Autodesk Inventor part; units mm, degrees
ref_plane "dummy_XY" through (0, 0, 0) normal (1, 0, 0) x (0, 0, -1)
ref_plane "dummy_YZ" through (0, 0, 0) normal (0, 0, -1) x (0, 1, 0)
ref_plane "dummy_ZX" through (0, 0, 0) normal (0, 1, 0) x (1, 0, 0)
sketch "Sketch_1" plane through (0, 0, 0) normal (1, 0, 0) x (0, 1, 0)
  line L0 (-22, 13) -> (-22.5, 12.5)
  line L1 (-22.5, 12.5) -> (-22.5, 2.25)
  line L2 (-22.5, 2.25) -> (-18.5, 2.25)
  line L3 (-18.5, 2.25) -> (-18.5, 1.9)
  arc A0 (-18.5, 1.9) -> (-18.3, 1.7) centre (-18.3, 1.9) ccw
  line L4 (-18.3, 1.7) -> (-17, 1.7)
  line L5 (-17, 1.7) -> (-16.5, 2.15)
  line L6 (-16.5, 2.15) -> (-14.7, 2.15)
  arc A1 (-13, 0.45) -> (-14.7, 2.15) centre (-14.7, 0.45) ccw
  line L7 (-13, 0.45) -> (-13, -0.45)
  arc A2 (-14.7, -2.15) -> (-13, -0.45) centre (-14.7, -0.45) ccw
  line L8 (-14.7, -2.15) -> (-16.5, -2.15)
  line L9 (-16.5, -2.15) -> (-17, -1.7)
  line L10 (-17, -1.7) -> (-18.3, -1.7)
  arc A3 (-18.3, -1.7) -> (-18.5, -1.9) centre (-18.3, -1.9) ccw
  line L11 (-18.5, -1.9) -> (-18.5, -2.25)
  line L12 (-18.5, -2.25) -> (-22.5, -2.25)
  line L13 (-22.5, -2.25) -> (-22.5, -12.5)
  line L14 (-22.5, -12.5) -> (-22, -13)
  line L15 (-22, -13) -> (22, -13)
  line L16 (22, -13) -> (22.5, -12.5)
  line L17 (22.5, -12.5) -> (22.5, -2.25)
  line L18 (22.5, -2.25) -> (18.5, -2.25)
  line L19 (18.5, -2.25) -> (18.5, -1.9)
  arc A4 (18.5, -1.9) -> (18.3, -1.7) centre (18.3, -1.9) ccw
  line L20 (18.3, -1.7) -> (17, -1.7)
  line L21 (17, -1.7) -> (16.5, -2.15)
  line L22 (16.5, -2.15) -> (14.7, -2.15)
  arc A5 (13, -0.45) -> (14.7, -2.15) centre (14.7, -0.45) ccw
  line L23 (13, -0.45) -> (13, 0.45)
  arc A6 (14.7, 2.15) -> (13, 0.45) centre (14.7, 0.45) ccw
  line L24 (14.7, 2.15) -> (16.5, 2.15)
  line L25 (16.5, 2.15) -> (17, 1.7)
  line L26 (17, 1.7) -> (18.3, 1.7)
  arc A7 (18.3, 1.7) -> (18.5, 1.9) centre (18.3, 1.9) ccw
  line L27 (18.5, 1.9) -> (18.5, 2.25)
  line L28 (18.5, 2.25) -> (22.5, 2.25)
  line L29 (22.5, 2.25) -> (22.5, 12.5)
  line L30 (22.5, 12.5) -> (22, 13)
  line L31 (22, 13) -> (-22, 13)
extrude "Extrusion1" add sketch "Sketch_1" along normal blind 50
sketch "Sketch2" plane through (50, 0, 0) normal (1, 0, 0) x (0, 0, -1)
  point P0 (0, 0)
hole "Hole1" at (50, 0, 0) direction (-1, 0, 0) diameter 22 depth 1.5
sketch "Sketch3" plane through (50, 0, 0) normal (1, 0, 0) x (0, 0, -1)
  point P0 (8, 17.5)
hole "Hole2" at (50, 17.5, -8) direction (-1, 0, 0) diameter 4 depth 4
sketch "Sketch_3" plane through (0, 0, 0) normal (0, 1, 0) x (-1, 0, 0)
  line L0 (0, 6.05) -> (-18.5, 6.05)
  line L1 (-18.5, 6.05) -> (-18.5, -6.05)
  line L2 (-18.5, -6.05) -> (0, -6.05)
  line L3 (0, -6.05) -> (0, 6.05)
extrude "Extrusion2" cut sketch "Sketch_3" along normal mid plane 60
sketch "Sketch5" plane through (50, 0, 0) normal (1, 0, 0) x (0, 0, -1)
  point P0 (8, -17.5)
hole "Hole3" at (50, -17.5, -8) direction (-1, 0, 0) diameter 4.134 depth 11 tip angle 120 countersink diameter 5 countersink angle 90
sketch "Sketch6" plane through (50, 0, 0) normal (1, 0, 0) x (0, 0, -1)
  point P0 (-8, 17.5)
hole "Hole4" at (50, 17.5, 8) direction (-1, 0, 0) diameter 4.134 depth 11 tip angle 120 countersink diameter 5 countersink angle 90
sketch "Sketch_6" plane through (0, 0, 6.5) normal (0, 0, 1) x (1, 0, 0)
  line L0 (25, 6.3066) -> (25, 22.5)
  line L1 (25, 22.5) -> (27.5, 22.5)
  line L2 (27.5, 22.5) -> (27.067, 22.067)
  line L3 (27.067, 22.067) -> (27.067, 15.5)
  line L4 (27.067, 15.5) -> (25.75, 14.7396)
  line L5 (25.75, 14.7396) -> (25.75, 6.7396)
  line L6 (25.75, 6.7396) -> (25, 6.3066)
  line L7 (25, 6.3066) -> (25, 22.5)
revolve "Revolution1" cut sketch "Sketch_6" angle 360 about axis through (25, 6.3066, 6.5) along (0, -1, 0)
thread "Thread1"
sketch "Sketch_7" plane through (0, 0, -6.5) normal (0, 0, 1) x (1, 0, 0)
  line L0 (42, 6.3066) -> (42, 22.5)
  line L1 (42, 22.5) -> (44.5, 22.5)
  line L2 (44.5, 22.5) -> (44.067, 22.067)
  line L3 (44.067, 22.067) -> (44.067, 15.5)
  line L4 (44.067, 15.5) -> (42.75, 14.7396)
  line L5 (42.75, 14.7396) -> (42.75, 6.7396)
  line L6 (42.75, 6.7396) -> (42, 6.3066)
  line L7 (42, 6.3066) -> (42, 22.5)
revolve "Revolution2" cut sketch "Sketch_7" angle 360 about axis through (42, 6.3066, -6.5) along (0, -1, 0)
thread "Thread2"
sketch "Sketch9" plane through (0, -22.5, 12.5) normal (0, -1, 0) x (1, 0, 0)
  point P0 (31, -4.5)
hole "Hole5" at (31, -22.5, 8) direction (0, 1, 0) diameter 4.134 depth 11 tip angle 120 countersink diameter 5 countersink angle 90
sketch "Sketch10" plane through (0, -22.5, -12.5) normal (0, -1, 0) x (1, 0, 0)
  point P0 (31, 4.5)
hole "Hole6" at (31, -22.5, -8) direction (0, 1, 0) diameter 4.134 depth 11 tip angle 120 countersink diameter 5 countersink angle 90
sketch "Sketch11" plane through (0, -22, -13) normal (0, 0, -1) x (-1, 0, 0)
  point P0 (-25, 7)
hole "Hole7" at (25, -15, -13) direction (0, 0, 1) diameter 4.134 depth 12 tip angle 120 countersink diameter 5 countersink angle 90
sketch "Sketch12" plane through (0, -22, -13) normal (0, 0, -1) x (-1, 0, 0)
  point P0 (-25, 37)
hole "Hole8" at (25, 15, -13) direction (0, 0, 1) diameter 4.134 depth 12 tip angle 120 countersink diameter 5 countersink angle 90
sketch "Sketch_14" plane through (0, 15, 0) normal (0, 1, 0) x (1, 0, 0)
  line L0 (10.5, -13) -> (10.5, 13)
  line L1 (10.5, 13) -> (12.7, 13)
  line L2 (12.7, 13) -> (12.5, 12.8)
  line L3 (12.5, 12.8) -> (12.5, -12.8)
  line L4 (12.5, -12.8) -> (12.7, -13)
  line L5 (12.7, -13) -> (10.5, -13)
  line L6 (10.5, -13) -> (10.5, 13)
revolve "Revolution3" cut sketch "Sketch_14" angle 360 about axis through (10.5, 15, 13) along (0, 0, 1)
sketch "Sketch_15" plane through (0, -15, 0) normal (0, 1, 0) x (1, 0, 0)
  line L0 (10.5, -13) -> (10.5, 13)
  line L1 (10.5, 13) -> (12.7, 13)
  line L2 (12.7, 13) -> (12.5, 12.8)
  line L3 (12.5, 12.8) -> (12.5, -12.8)
  line L4 (12.5, -12.8) -> (12.7, -13)
  line L5 (12.7, -13) -> (10.5, -13)
  line L6 (10.5, -13) -> (10.5, 13)
revolve "Revolution4" cut sketch "Sketch_15" angle 360 about axis through (10.5, -15, 13) along (0, 0, 1)
sketch "Sketch_20" plane through (10.5, 0, 0) normal (1, 0, 0) x (0, 0, -1)
  line L0 (-12.9, 15) -> (12.9, 15)
  line L1 (12.9, 15) -> (12.9, 13)
  line L2 (12.9, 13) -> (-12.9, 13)
  line L3 (-12.9, 13) -> (-12.9, 15)
  line L4 (-12.9, 15) -> (12.9, 15)
revolve "Revolution5" add sketch "Sketch_20" angle 360 about axis through (10.5, 15, 12.9) along (0, 0, 1)
sketch "Sketch_21" plane through (10.5, 0, 0) normal (1, 0, 0) x (0, 0, -1)
  line L0 (-12.9, -15) -> (12.9, -15)
  line L1 (12.9, -15) -> (12.9, -17)
  line L2 (12.9, -17) -> (-12.9, -17)
  line L3 (-12.9, -17) -> (-12.9, -15)
  line L4 (-12.9, -15) -> (12.9, -15)
revolve "Revolution6" add sketch "Sketch_21" angle 360 about axis through (10.5, -15, 12.9) along (0, 0, 1)
ref_plane "dummy_XY" through (0, 0, 0) normal (1, 0, 0) x (0, 0, -1)
ref_plane "dummy_YZ" through (0, 0, 0) normal (0, 0, -1) x (0, 1, 0)
ref_plane "dummy_ZX" through (0, 0, 0) normal (0, 1, 0) x (1, 0, 0)
ref_plane "grip_XY" through (10.5, 15, 0) normal (0, 0, 1) x (1, 0, 0)
ref_plane "grip_YZ" through (10.5, 15, 0) normal (1, 0, 0) x (0, 1, 0)
ref_plane "grip_ZX" through (10.5, 15, 0) normal (0, 1, 0) x (0, 0, 1)
ref_plane "grip1_XY" through (10.5, -15, 0) normal (0, 0, 1) x (1, 0, 0)
ref_plane "grip1_YZ" through (10.5, -15, 0) normal (1, 0, 0) x (0, 1, 0)
ref_plane "grip1_ZX" through (10.5, -15, 0) normal (0, 1, 0) x (0, 0, 1)
ref_plane "switch_XY" through (20.8, 13, 0) normal (-1, 0, 0) x (0, 0, -1)
ref_plane "switch_YZ" through (20.8, 13, 0) normal (0, 0, -1) x (0, -1, 0)
ref_plane "switch_ZX" through (20.8, 13, 0) normal (0, -1, 0) x (-1, 0, 0)
ref_plane "switch2_XY" through (26.1, -13, 0) normal (-1, 0, 0) x (0, 0, -1)
ref_plane "switch2_YZ" through (26.1, -13, 0) normal (0, 0, -1) x (0, -1, 0)
ref_plane "switch2_ZX" through (26.1, -13, 0) normal (0, -1, 0) x (-1, 0, 0)
properties part number "MCHA-20_(b)"
For this review, take the finished solid that the model builds, in its own axes (mm). A direction names the side the tool comes from. Round coordinates to 2 decimals unless told otherwise and drop trailing zeros. Write each loop counter-clockwise with the first axis right and the second up, starting at its lowest first coordinate (ties: lowest second). Pieces come first, ordered by that corner, then holes. Notation, with made-up numbers: (-26.5, 40.25) -> (8.5, 40.25) arc R8 ccw to (8.5, 51.25) -> close; hole circle Ø3 at (75.25, 7.5). An arc over 180 degrees is marked (long way). Use CSV: the item, a comma, the result in double quotes.
(1) Consider section A-A, the plane y = 3. Give the boundary of the cut face in (x, z), plus the area to 3 significant figures.
Computed values:
outline,"(0, -13) -> (50, -13) -> (50, -10.58) -> (48.5, -10.58) -> (48.5, 10.58) -> (50, 10.58) -> (50, 13) -> (0, 13) -> (0, 6.05) -> (18.5, 6.05) -> (18.5, -6.05) -> (0, -6.05) -> close"
area,"1,040 mm²"
(2) Clearance check with flat-ended pins moving along their axes: P1, Ø11, axis at y = 3, z = -5, coming from the +X side; P2, Ø1.2, axis at x = 10, y = 14.5, coming from the +Z side; P3, Ø1.2, axis at x = 10.5, y = -15, coming from the -Z side; P4, Ø0.5, axis at x = 29, z = 0, coming from the -Y side. State where each tip first meets the part, or that it passes through.
Computed values:
P1,"x = 50"
P2,"z = 12.9"
P3,"z = -12.9"
P4,"y = -13"
(3) To check wall thickness, follow L1, parallel to Y at x = 25, z = -8.5; L2, parallel to Z at x = 31, y = -17; L3, parallel to Y at x = 45, z = 8. State the ranges of each line that lie inside material, in increasing order. Write a range as [from, to].
Computed values:
L1,"[-22.5, -17.07], [-12.93, 12.93], [17.07, 22.5]"
L2,"[-13, -10.07], [-5.93, -1.7], [1.7, 5.93], [10.07, 13]"
L3,"[-22.5, 15.43], [19.57, 22.5]"
(4) Draft analysis for pull direction X (two halves, no side actions). For faces 1 (the face through (38.01, -17.26, -7.74)), 2 (the face through (34, 18, 1.7)), 3 (the face through (24.38, -13.03, -6.7)), state which applies: +X half, -X half, draft (parallel to the pull), parting line (faces both ways), or undercut.
Computed values:
face 1,"+X half"
face 2,"draft"
face 3,"undercut"
(5) For faces 4 (the face through (26.97, 18.74, 7.12)), 5 (the face through (34, 16, 2.15)), 6 (the face through (18.5, 0, 0)), 7 (the face through (34, -21, 2.25)), 8 (the face through (25, 0, 13)), list the 3-axis set-ups (+Z, -Z, +X, -X, +Y, -Y) from which the entire face can be reached by the end or side of a thin tool; tool diameter is ignored.
Computed values:
face 4,"+Y"
face 5,"+X"
face 6,"+Y, -Y"
face 7,"+X, -X, -Y"
face 8,"+Z, +X, -X, +Y, -Y"
